For this review, take the finished solid that the model builds, in its own axes (mm). A direction names the side the tool comes from. Give positions to 0.01 mm unless a question says otherwise; leave off trailing zeros. Loops run counter-clockwise (first coordinate to the right, second up) from the corner with the lowest first, then second, coordinate; pieces in that order, holes last. Notation, with made-up numbers: (-15, 31.25) - (2, 31.25) arc R16 cw to (2, 48.25) - close; hole circle Ø1 at (-22, 33.25). An arc over 180 degrees is marked (long way). Answer in a Markdown table with one row per item.
```python
from build123d import *

# Parameters (mm, degrees)
F0_W     = 85.725
F0_H     = 6.35
F1_DEPTH = 6.35
F2_W     = 6.35
F2_H     = 22.225
F3_DEPTH = 4.7625
F4_W     = 6.35
F4_H     = 6.35
F5_DEPTH = 38.1


with BuildPart() as f1:
    # F0 (on Front) → F1 (new body)
    with BuildSketch(Plane.XZ):
        with Locations((-2.977964, 37.027801)):
            Rectangle(F0_W, F0_H)
    extrude(amount=F1_DEPTH)

    # F2 (on face) → F3 (join)
    with BuildSketch(Plane(origin=(-45.840464, 0, 0), x_dir=(0, -1, 0), z_dir=(-1, 0, 0))):
        with Locations((3.175, 44.965301)):
            Rectangle(F2_W, F2_H)
    extrude(amount=-F3_DEPTH)

    # F4 (on face) → F5 (join)
    with BuildSketch(Plane(origin=(0, 0, 33.852801), x_dir=(1, 0, 0), z_dir=(0, 0, -1))):
        with Locations((-4.565464, 3.175)):
            Rectangle(F4_W, F4_H)
    extrude(amount=F5_DEPTH)


solid = f1.part
```
1. Clearance check with flat-ended pins moving along their axes: pin 1 (1.5 mm diameter, centred on x = 3.5, y = -1.5, fed in from -Z); pin 2 (1.9 mm diameter, centred on y = -3, z = 6.5, fed in from +X); pin 3 (2 mm diameter, centred on y = -5.5, z = 43.5, fed in from +X). State where each tip first meets the part, or that it passes through.
Values:
| item | result |
|---|---|
| pin 1 | stops at z = 33.85 |
| pin 2 | stops at x = -1.39 |
| pin 3 | stops at x = -41.08 |
2. We need section B-B, the plane x = -27.5. Give the boundary of the cut face in (y, z), and give its area (3 significant figures).
Values:
| item | result |
|---|---|
| outline | (-6.35, 33.85) - (0, 33.85) - (0, 40.2) - (-6.35, 40.2) - close |
| area | 40.3 mm^2 |
3. We need section A-A, the plane y = -5.5. Give the boundary of the cut face in (x, z), and give its area (3 significant figures).
Values:
| item | result |
|---|---|
| outline | (-45.84, 33.85) - (-7.74, 33.85) - (-7.74, -4.25) - (-1.39, -4.25) - (-1.39, 33.85) - (39.88, 33.85) - (39.88, 40.2) - (-41.08, 40.2) - (-41.08, 56.08) - (-45.84, 56.08) - close |
| area | 862 mm^2 |
4. Wall thickness on line 1 (X direction, y = -4.75, z = 4); line 2 (Z direction, x = 1, y = -0.75); line 3 (Z direction, x = -2, y = -1.5): over which ranges is each line inside the solid? List them lowest first. Write a range as [from, to].
Values:
| item | result |
|---|---|
| line 1 | x = [-7.74, -1.39] |
| line 2 | z = [33.85, 40.2] |
| line 3 | z = [-4.25, 40.2] |
5. Mouldability with a two-part tool opening along X and no side actions: class faces 5 (the face through (-45.84, -3, 45)), 6 (the face through (-43, -3, 56.078)), 7 (the face through (-41.078, -3, 48)) as released by +X, released by -X, zero draft, split by the parting line, or undercut.
Values:
| item | result |
|---|---|
| face 5 | released by -X |
| face 6 | zero draft |
| face 7 | released by +X |
6. We need section C-C, the plane z = 47. Give the boundary of the cut face in (x, y).
Values:
| item | result |
|---|---|
| outline | (-45.84, -6.35) - (-41.08, -6.35) - (-41.08, 0) - (-45.84, 0) - close |
7. For faces 1 (the face through (-1, -3, 40.203)), 2 (the face through (-27, -3, 33.853)), 3 (the face through (-1.39, -3, 15)), 4 (the face through (39.885, -3, 37)), list the 3-axis set-ups (+Z, -Z, +X, -X, +Y, -Y) from which the entire face can be reached by the end or side of a thin tool; tool diameter is ignored.
Values:
| item | result |
|---|---|
| face 1 | +Z, +X, +Y, -Y |
| face 2 | -Z, -X, +Y, -Y |
| face 3 | -Z, +X, +Y, -Y |
| face 4 | +Z, -Z, +X, +Y, -Y |
